Build history of the part. All positions in model axes, mm. Give positions to 0.01 mm unless a question says otherwise; leave off trailing zeros. Order: outer loops, then holes, each group sorted by start corner. A loop starts at its lowest first (then second) coordinate and runs counter-clockwise, first axis right, second up. Notation, with made-up numbers: (-9, 50) - (10, 50) arc R18 ccw to (10, 84) - close; hole circle Ø3 at (-4, 35). An arc over 180 degrees is marked (long way). Write each question's results on one line, items separated by ' | '. Start each with the question number.
1) Drill centre lines: line 1 along X through (y, z) = (4.75, 14.5); line 2 along Y through (x, z) = (5.25, 13.5); line 3 along Z through (x, y) = (1.75, 0.5). Where is each one in solid material? Low to high. Write a range as from..to.
2) Cut at B-B on y = -1.5. List the corners of the cut face in (x, z), plus the area to 3 significant figures.
3) Drop flat-ended pins along their axis: pin 1 Ø1.5 at (x, y) = (1.5, -1) entering from -Z (3 decimals); pin 2 Ø3 at (x, y) = (4.5, -4) entering from -Z; pin 3 Ø3 at (x, y) = (-7.5, -7) entering from -Z. Give the stop position or say it passes through.
4) Cut at C-C on x = 4.5. List the corners of the cut face in (y, z).
5) Cut at A-A on z = 9. List the corners of the cut face in (x, y).
6) Cut at D-D on z = 11.75. List the corners of the cut face in (x, y), plus the area to 3 significant figures.
from build123d import *

# Parameters (mm, degrees)
SKETCH1_R           = 10
BOSS_EXTRUDE1_DEPTH = 15
CUT_EXTRUDE1_DEPTH  = 16
CUT_EXTRUDE2_DEPTH  = 10
CUT_EXTRUDE3_DEPTH  = 10
SKETCH7_W           = 15
SKETCH7_H           = 10
BOSS_EXTRUDE2_DEPTH = 10
CUT_EXTRUDE4_DEPTH  = 20


with BuildPart() as part:
    # Sketch1 → Boss-Extrude1 (new body)
    with BuildSketch(Plane.XY):
        Circle(SKETCH1_R)
    extrude(amount=BOSS_EXTRUDE1_DEPTH)

    # Sketch2 → Cut-Extrude1 (cut, through all)
    with BuildSketch(Plane.XY.offset(15)):
        with BuildLine():
            Line((0, 0), (10, 0))
            ThreePointArc((10, 0), (7.071067812, -7.071067812), (0, -10))
            Line((0, -10), (0, 0))
        make_face()
    extrude(amount=-CUT_EXTRUDE1_DEPTH, mode=Mode.SUBTRACT)

    # Sketch5 → Cut-Extrude2 (cut)
    with BuildSketch(Plane(origin=(10, 0, 0), x_dir=(0, 0, -1), z_dir=(1, 0, 0))):
        Polygon((0, 0), (0, 10), (-15, 10), align=None)
    extrude(amount=-CUT_EXTRUDE2_DEPTH, mode=Mode.SUBTRACT)

    # Sketch6 → Cut-Extrude3 (cut)
    with BuildSketch(Plane(origin=(0, 0, 0), x_dir=(0, 0, -1), z_dir=(1, 0, 0))):
        Polygon((-15, 10), (0, 0), (0, 10), align=None)
    extrude(amount=-CUT_EXTRUDE3_DEPTH, mode=Mode.SUBTRACT)

    # Sketch7 → Boss-Extrude2 (add, symmetric)
    with BuildSketch(Plane(origin=(0, 0, 0), x_dir=(0, 0, -1), z_dir=(1, 0, 0))):
        with Locations((-7.5, -5)):
            Rectangle(SKETCH7_W, SKETCH7_H)
    extrude(amount=BOSS_EXTRUDE2_DEPTH, both=True)

    # Sketch8 → Cut-Extrude4 (cut)
    with BuildSketch(Plane(origin=(10, 0, 0), x_dir=(0, 0, -1), z_dir=(1, 0, 0))):
        Polygon((0, 0), (-15, -10), (0, -10), align=None)
    extrude(amount=-CUT_EXTRUDE4_DEPTH, mode=Mode.SUBTRACT)


solid = part.part
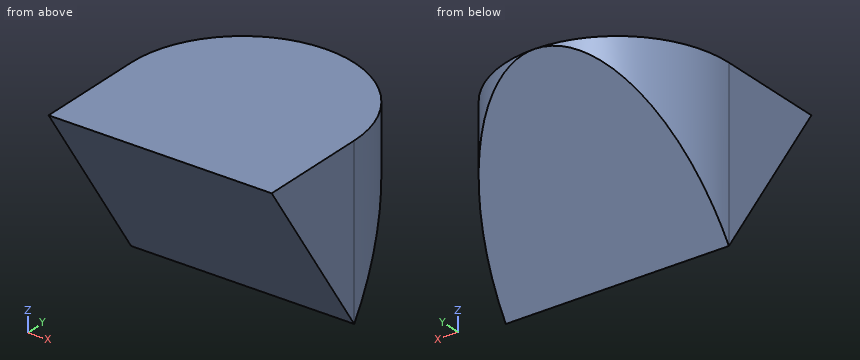
Results:
1) line 1: -8.8..8.8 | line 2: -9..8.51 | line 3: 0.75..15
2) outline: (-10, 2.25) - (10, 2.25) - (10, 15) - (-10, 15) - close | area: 255 mm^2
3) pin 1: z = 0.375 | pin 2: z = 3.75 | pin 3: z = 8.25
4) outline: (-10, 15) - (0, 0) - (8.93, 13.4) - (8.93, 15) - close
5) outline: (-10, -6) - (10, -6) - (10, 0) arc R10 ccw to (8, 6) - (-8, 6) arc R10 ccw to (-10, 0) - close
6) outline: (-10, -7.83) - (10, -7.83) - (10, 0) arc R10 ccw to (6.22, 7.83) - (-6.22, 7.83) arc R10 ccw to (-10, 0) - close | area: 295 mm^2
